CAD build for the part. Positions are in the model's coordinates, mm. A direction names the side the tool comes from. Round coordinates to 2 decimals unless told otherwise and drop trailing zeros. Order: outer loops, then holes, each group sorted by start corner. A loop starts at its lowest first (then second) coordinate and runs counter-clockwise, first axis right, second up. Notation, with made-up numbers: (33.5, -21.5) - (83.5, -21.5) arc R22 ccw to (83.5, 17.5) - close; hole circle Ø5 at (-33, -10.75). An arc over 180 degrees is marked (long way). Write item = value, one per line.
from build123d import *
from build123d.topology import SkipClean

# Parameters (mm, degrees)
SKETCH1_W                                           = 73
SKETCH1_H                                           = 12
SKETCH1_R                                           = 2.5
BOSS_EXTRUDE1_DEPTH                                 = 2.5
FILLET1_R                                           = 5
CHAMFER1_SIZE                                       = 0.75
CHAMFER1_SIZE_2                                     = 0.534818385
CSK_FOR_M3_COUNTERSUNK_FLAT_HEAD_SCREW1_D           = 3.2
CSK_FOR_M3_COUNTERSUNK_FLAT_HEAD_SCREW1_CSINK_D     = 6.3
CSK_FOR_M3_COUNTERSUNK_FLAT_HEAD_SCREW1_CSINK_ANGLE = 90
CUT_EXTRUDE1_DEPTH                                  = 1.25


with BuildPart() as part:
    # Sketch1 → Boss-Extrude1 (new, symmetric)
    with BuildSketch(Plane.XY):
        Rectangle(SKETCH1_W, SKETCH1_H)
        with Locations((-30.5, 0)):
            Circle(SKETCH1_R, mode=Mode.SUBTRACT)
        with Locations((30.5, 0)):
            Circle(SKETCH1_R, mode=Mode.SUBTRACT)
    extrude(amount=BOSS_EXTRUDE1_DEPTH, both=True)

    # Sketch2 → Cut-Revolve1 (revolve, cut)
    with SkipClean():  # the faces are left unmerged after this step: merging them gives an invalid solid
        with BuildSketch(Plane(origin=(0, 0, 0), x_dir=(1, 0, 0), z_dir=(0, 1, 0)), mode=Mode.PRIVATE) as cut_revolve1_sk:
            with BuildLine():
                ThreePointArc((-30.5, 4.1), (-34.6, 0), (-30.5, -4.1))
                Line((-30.5, -4.1), (-30.5, 4.1))
            make_face()
            with BuildLine():
                Line((-30.5, 4.1), (-30.5, -4.1))
                ThreePointArc((-30.5, -4.1), (-27.600862197, -2.899137803), (-26.4, 0))
                ThreePointArc((-26.4, 0), (-27.600862197, 2.899137803), (-30.5, 4.1))
            make_face()
        cut_revolve1 = revolve(cut_revolve1_sk.sketch.rotate(Axis((-30.5, 0, 14.750329737), (0, 0, -1)), 180), axis=Axis((-30.5, 0, 14.750329737), (0, 0, -1)), mode=Mode.SUBTRACT)
    add(part.part.scale(1), mode=Mode.REPLACE)  # the faces are merged on a copy

    # Mirror1: Cut-Revolve1 across plane
    add(cut_revolve1.mirror(Plane(origin=(0, 0, 0), x_dir=(0, 0, 1), z_dir=(1, 0, 0))), mode=Mode.SUBTRACT)

    # Fillet1
    fillet1_edges = [part.edges().sort_by_distance(p)[0] for p in [
        (36.5, -6, 0),
        (-36.5, -6, 0),
        (-36.5, 6, 0),
        (36.5, 6, 0),
    ]]
    fillet(fillet1_edges, radius=FILLET1_R)

    # Chamfer1
    # the kernel refuses this chamfer: 0.75, 0.534818385 mm, written as the material it takes off along each edge
    with BuildSketch(Plane(origin=(-30.5, 0, 2.5), x_dir=(1, 0, 0), z_dir=(0, -1, 0))) as chamfer1_piece_1:
        with BuildLine():
            Line((3.249615362 + CHAMFER1_SIZE, 0), (3.550305573, -0.449309789))
            ThreePointArc((3.550305573, -0.449309789), (3.409004663, -0.222130994), (3.249615362, 0))
            Line((3.249615362, 0), (3.249615362 + CHAMFER1_SIZE, 0))
        make_face()
    revolve(axis=Axis((-30.5, 0, 2.5), (0, 0, 1)), mode=Mode.SUBTRACT)
    with BuildSketch(Plane(origin=(30.5, 0, 2.5), x_dir=(-1, 0, 0), z_dir=(0, 1, 0))) as chamfer1_piece_2:
        with BuildLine():
            Line((3.249615362 + CHAMFER1_SIZE, 0), (3.550305573, -0.449309789))
            ThreePointArc((3.550305573, -0.449309789), (3.409004663, -0.222130994), (3.249615362, 0))
            Line((3.249615362, 0), (3.249615362 + CHAMFER1_SIZE, 0))
        make_face()
    revolve(axis=Axis((30.5, 0, 2.5), (0, 0, 1)), mode=Mode.SUBTRACT)
    with BuildSketch(Plane(origin=(-30.5, 0, -2.5), x_dir=(1, 0, 0), z_dir=(0, -1, 0))) as chamfer1_piece_3:
        with BuildLine():
            Line((3.249615362 + CHAMFER1_SIZE_2, 0), (3.691177382, 0.715284467))
            ThreePointArc((3.691177382, 0.715284467), (3.494921898, 0.356283384), (3.249615362, 0))
            Line((3.249615362, 0), (3.249615362 + CHAMFER1_SIZE_2, 0))
        make_face()
    revolve(axis=Axis((-30.5, 0, -2.5), (0, 0, 1)), mode=Mode.SUBTRACT)
    with BuildSketch(Plane(origin=(30.5, 0, -2.5), x_dir=(-1, 0, 0), z_dir=(0, 1, 0))) as chamfer1_piece_4:
        with BuildLine():
            Line((3.249615362 + CHAMFER1_SIZE_2, 0), (3.691177382, 0.715284467))
            ThreePointArc((3.691177382, 0.715284467), (3.494921898, 0.356283384), (3.249615362, 0))
            Line((3.249615362, 0), (3.249615362 + CHAMFER1_SIZE_2, 0))
        make_face()
    revolve(axis=Axis((30.5, 0, -2.5), (0, 0, 1)), mode=Mode.SUBTRACT)
    with BuildSketch(Plane(origin=(-31.5, 6, -2.5), x_dir=(0, 0, 1), z_dir=(1, 0, 0)), Plane(origin=(31.5, -6, 2.5), x_dir=(0, 1, 0), z_dir=(-1, 0, 0))) as chamfer1_piece_5:
        Polygon((CHAMFER1_SIZE, 0), (0, CHAMFER1_SIZE), (0, 0), align=None)
    extrude(amount=63, mode=Mode.SUBTRACT)
    with BuildSketch(Plane(origin=(-31.5, 6, 2.5), x_dir=(0, 0, -1), z_dir=(1, 0, 0)), Plane(origin=(31.5, -6, -2.5), x_dir=(0, 1, 0), z_dir=(-1, 0, 0))) as chamfer1_piece_6:
        Polygon((CHAMFER1_SIZE, 0), (0, -CHAMFER1_SIZE), (0, 0), align=None)
    extrude(amount=63, mode=Mode.SUBTRACT)
    with BuildSketch(Plane(origin=(36.5, 1, -2.5), x_dir=(-1, 0, 0), z_dir=(0, -1, 0)), Plane(origin=(-36.5, -1, -2.5), x_dir=(1, 0, 0), z_dir=(0, 1, 0))) as chamfer1_piece_7:
        Polygon((CHAMFER1_SIZE, 0), (0, -CHAMFER1_SIZE), (0, 0), align=None)
    extrude(amount=2, mode=Mode.SUBTRACT)
    with BuildSketch(Plane(origin=(-31.5, -1, -2.5), x_dir=(-1, 0, 0), z_dir=(0, 1, 0))) as chamfer1_piece_8:
        Polygon((5 - CHAMFER1_SIZE, 0), (5, CHAMFER1_SIZE), (5, 0), align=None)
    revolve(axis=Axis((-31.5, -1, -2.5), (0, 0, 1)), revolution_arc=90, mode=Mode.SUBTRACT)
    with BuildSketch(Plane(origin=(-31.5, 1, -2.5), x_dir=(0, 1, 0), z_dir=(1, 0, 0))) as chamfer1_piece_9:
        Polygon((5 - CHAMFER1_SIZE, 0), (5, CHAMFER1_SIZE), (5, 0), align=None)
    revolve(axis=Axis((-31.5, 1, -2.5), (0, 0, 1)), revolution_arc=90, mode=Mode.SUBTRACT)
    with BuildSketch(Plane(origin=(31.5, -1, -2.5), x_dir=(1, 0, 0), z_dir=(0, 1, 0))) as chamfer1_piece_10:
        Polygon((5 - CHAMFER1_SIZE, 0), (5, -CHAMFER1_SIZE), (5, 0), align=None)
    revolve(axis=Axis((31.5, -1, -2.5), (0, 0, -1)), revolution_arc=90, mode=Mode.SUBTRACT)
    with BuildSketch(Plane(origin=(31.5, 1, -2.5), x_dir=(0, 1, 0), z_dir=(-1, 0, 0))) as chamfer1_piece_11:
        Polygon((5 - CHAMFER1_SIZE, 0), (5, -CHAMFER1_SIZE), (5, 0), align=None)
    revolve(axis=Axis((31.5, 1, -2.5), (0, 0, -1)), revolution_arc=90, mode=Mode.SUBTRACT)
    with BuildSketch(Plane(origin=(36.5, 1, 2.5), x_dir=(-1, 0, 0), z_dir=(0, -1, 0)), Plane(origin=(-36.5, -1, 2.5), x_dir=(1, 0, 0), z_dir=(0, 1, 0))) as chamfer1_piece_12:
        Polygon((CHAMFER1_SIZE, 0), (0, CHAMFER1_SIZE), (0, 0), align=None)
    extrude(amount=2, mode=Mode.SUBTRACT)
    with BuildSketch(Plane(origin=(-31.5, -1, 2.5), x_dir=(-1, 0, 0), z_dir=(0, 1, 0))) as chamfer1_piece_13:
        Polygon((5 - CHAMFER1_SIZE, 0), (5, -CHAMFER1_SIZE), (5, 0), align=None)
    revolve(axis=Axis((-31.5, -1, 2.5), (0, 0, 1)), revolution_arc=90, mode=Mode.SUBTRACT)
    with BuildSketch(Plane(origin=(-31.5, 1, 2.5), x_dir=(0, 1, 0), z_dir=(1, 0, 0))) as chamfer1_piece_14:
        Polygon((5, -CHAMFER1_SIZE), (5 - CHAMFER1_SIZE, 0), (5, 0), align=None)
    revolve(axis=Axis((-31.5, 1, 2.5), (0, 0, 1)), revolution_arc=90, mode=Mode.SUBTRACT)
    with BuildSketch(Plane(origin=(31.5, -1, 2.5), x_dir=(1, 0, 0), z_dir=(0, 1, 0))) as chamfer1_piece_15:
        Polygon((5 - CHAMFER1_SIZE, 0), (5, CHAMFER1_SIZE), (5, 0), align=None)
    revolve(axis=Axis((31.5, -1, 2.5), (0, 0, -1)), revolution_arc=90, mode=Mode.SUBTRACT)
    with BuildSketch(Plane(origin=(31.5, 1, 2.5), x_dir=(0, 1, 0), z_dir=(-1, 0, 0))) as chamfer1_piece_16:
        Polygon((5, CHAMFER1_SIZE), (5 - CHAMFER1_SIZE, 0), (5, 0), align=None)
    revolve(axis=Axis((31.5, 1, 2.5), (0, 0, -1)), revolution_arc=90, mode=Mode.SUBTRACT)

    # CSK for M3 Countersunk Flat Head Screw1 (through all)
    with Locations(Plane(origin=(0, 0, -2.5), x_dir=(-1, 0, 0), z_dir=(0, 0, -1))):
        with Locations((-22.5, 0), (22.5, 0)):
            CounterSinkHole(CSK_FOR_M3_COUNTERSUNK_FLAT_HEAD_SCREW1_D / 2, CSK_FOR_M3_COUNTERSUNK_FLAT_HEAD_SCREW1_CSINK_D / 2, counter_sink_angle=CSK_FOR_M3_COUNTERSUNK_FLAT_HEAD_SCREW1_CSINK_ANGLE)

    # Sketch6 → Cut-Extrude1 (cut)
    with BuildSketch(Plane.XY.offset(2.5)):
        Polygon((-19.209103466, 0), (-20.854551733, 2.85), (-24.145448267, 2.85), (-25.790896534, 0), (-24.145448267, -2.85), (-20.854551733, -2.85), align=None)
        Polygon((19.209103466, 0), (20.854551733, -2.85), (24.145448267, -2.85), (25.790896534, 0), (24.145448267, 2.85), (20.854551733, 2.85), align=None)
    extrude(amount=-CUT_EXTRUDE1_DEPTH, mode=Mode.SUBTRACT)


solid = part.part
(1) Probe line 1 along X through (y, z) = (2.5, -1.2); line 2 along Y through (x, z) = (-22.5, -0.05); line 3 along X through (y, z) = (-3.5, 0.35). List the from-to ranges inside material, lowest first.
Solved:
line_1 = -36.27 to -33.52, -27.48 to 27.48, 33.52 to 36.27
line_2 = -6 to -1.6, 1.6 to 6
line_3 = -35.83 to -32.61, -28.39 to 28.39, 32.61 to 35.83
(2) Band-saw the part on C-C on x = -9. List the corners of the cut face in (y, z).
Solved:
outline = (-6, -1.75) - (-5.25, -2.5) - (5.25, -2.5) - (6, -1.75) - (6, 1.75) - (5.25, 2.5) - (-5.25, 2.5) - (-6, 1.75) - close
(3) Pull direction Y, two halves, no side cores. Call faces 1 (the flat face through (-1, 0, 2.5)), 2 (the conical face through (-34.56, 4.12, 2.38)), 3 (the flat face through (-22, 2.85, 2)), 4 (the cylindrical face through (24.026, 0.481, 0.165)): released by +Y, released by -Y, zero draft, split by the parting line, or undercut.
Solved:
face_1 = zero draft
face_2 = released by +Y
face_3 = undercut
face_4 = undercut
(4) Drop flat-ended pins along their axis: pin 1 (1.7 mm diameter, centred on x = -22.5, y = -1.5, fed in from +Z); pin 2 (1 mm diameter, centred on y = -1.5, z = 1.5, fed in from -X); pin 3 (4 mm diameter, centred on x = -22.5, y = 0, fed in from -Z); pin 4 (1 mm diameter, centred on y = 4, z = -2, fed in from +X). Give the stop position or say it passes through.
Solved:
pin_1 = 1.25
pin_2 = -36.5
pin_3 = -1.35
pin_4 = 35.79
(5) Band-saw the part on A-A on x = -22.5. List the corners of the cut face in (y, z), plus the area to 3 significant figures.
Solved:
outline = (-6, -1.75) - (-5.25, -2.5) - (-3.15, -2.5) - (-1.6, -0.95) - (-1.6, 1.25) - (-2.85, 1.25) - (-2.85, 2.5) - (-5.25, 2.5) - (-6, 1.75) - close; (1.6, -0.95) - (3.15, -2.5) - (5.25, -2.5) - (6, -1.75) - (6, 1.75) - (5.25, 2.5) - (2.85, 2.5) - (2.85, 1.25) - (1.6, 1.25) - close
area = 37.3 mm²
(6) Band-saw the part on B-B on z = -0.1. List the corners of the cut face in (x, y).
Solved:
outline = (-36.5, -1) arc R5 ccw to (-31.5, -6) - (31.5, -6) arc R5 ccw to (36.5, -1) - (36.5, 1) arc R5 ccw to (31.5, 6) - (-31.5, 6) arc R5 ccw to (-36.5, 1) - close; hole circle Ø8.2 at (-30.5, 0); hole circle Ø3.2 at (-22.5, 0); hole circle Ø3.2 at (22.5, 0); hole circle Ø8.2 at (30.5, 0)
(7) Tool access for faces 5 (the cylindrical face through (35.07, -4.5, 0.02)), 6 (the flat face through (-23, -2.85, 2)): list every direction of +Z, -Z, +X, -X, +Y, -Y with a clear straight run to the whole face (end or side of a thin tool).
Solved:
face_5 = +Z, -Z, +X, -Y
face_6 = +Z
(8) Band-saw the part on D-D on x = 30.5. List the corners of the cut face in (y, z), plus the area to 3 significant figures.
Solved:
outline = (-6, -1.75) - (-5.25, -2.5) - (-3.78, -2.5) - (-3.69, -1.78) arc R4.1 cw to (-3.55, 2.05) - (-4, 2.5) - (-5.25, 2.5) - (-6, 1.75) - close; (3.55, 2.05) arc R4.1 cw to (3.69, -1.78) - (3.78, -2.5) - (5.25, -2.5) - (6, -1.75) - (6, 1.75) - (5.25, 2.5) - (4, 2.5) - close
area = 19.9 mm²
